```python
from build123d import *

# Parameters (mm, degrees)
F0_R     = 2.65
F0_R_2   = 3.15
F1_DEPTH = 5
F2_R     = 4
F3_R     = 3


with BuildPart() as f1:
    # F0 (on Top) → F1 (new body)
    with BuildSketch(Plane.XY):
        with BuildLine():
            ThreePointArc((-30, -20), (0, -14.852814), (30, -20))
            ThreePointArc((30, -20), (26.568542, 0), (30, 20))
            ThreePointArc((30, 20), (0, 14.852814), (-30, 20))
            ThreePointArc((-30, 20), (-26.568542, 0), (-30, -20))
        make_face()
        with Locations((-20, -10)):
            Circle(F0_R, mode=Mode.SUBTRACT)
        with Locations((20, -10)):
            Circle(F0_R, mode=Mode.SUBTRACT)
        with Locations((-20, 10)):
            Circle(F0_R_2, mode=Mode.SUBTRACT)
        Polygon((10, 0), (5, -8.660254), (-5, -8.660254), (-10, 0), (-5, 8.660254), (5, 8.660254), align=None, mode=Mode.SUBTRACT)
        with Locations((20, 10)):
            Circle(F0_R_2, mode=Mode.SUBTRACT)
    extrude(amount=F1_DEPTH)

    # F2
    f2_edges = [f1.edges().sort_by_distance(p)[0] for p in [
        (30, 20, 2.5),
        (-30, 20, 2.5),
        (-30, -20, 2.5),
        (30, -20, 2.5),
    ]]
    fillet(f2_edges, radius=F2_R)

    # F3
    f3_edges = [f1.edges().sort_by_distance(p)[0] for p in [
        (5, 8.660254, 2.5),
        (-5, 8.660254, 2.5),
        (10, 0, 2.5),
        (5, -8.660254, 2.5),
        (-5, -8.660254, 2.5),
        (-10, 0, 2.5),
    ]]
    fillet(f3_edges, radius=F3_R)


solid = f1.part
```
Verification items for the finished model (mm, model axes). A direction names the side the tool comes from. Coordinates: 2 decimals unless noted, no trailing zeros. Write each loop counter-clockwise with the first axis right and the second up, starting at its lowest first coordinate (ties: lowest second). Pieces come first, ordered by that corner, then holes. Notation, with made-up numbers: M 83.25,-17.75 L 115.25,-17.75 A15 cw 115.25,2.25 Z; hole C 17.25,73.5 d1. An arc over 180 degrees is marked long. One line per item, written item: value.
Item 1: Section check A-A, the plane x = -4. Record the boundary of the cut face in (y, z).
Check sheet entries:
outline: M -14.94,0 L -8.57,0 L -8.57,5 L -14.94,5 Z; M 8.57,0 L 14.94,0 L 14.94,5 L 8.57,5 Z
Item 2: Mould release check, pull along Y, two halves, no side actions. Record for faces 3 (the cylindrical face through (0.327, 14.853, 2.465)), 4 (the cylindrical face through (-4.75, -8.27, 2.54)), 5 (the flat face through (6, -8, 5)): pulls with the +Y half, pulls with the -Y half, needs draft (parallel to the pull), parting line crosses it, or undercut.
Check sheet entries:
face 3: pulls with the +Y half
face 4: undercut
face 5: needs draft
Item 3: Section check D-D, the plane x = 21.5. Record the boundary of the cut face in (y, z).
Check sheet entries:
outline: M -17.46,0 L -12.18,0 L -12.18,5 L -17.46,5 Z; M -7.82,0 L 7.23,0 L 7.23,5 L -7.82,5 Z; M 12.77,0 L 17.46,0 L 17.46,5 L 12.77,5 Z
Item 4: Section check C-C, the plane y = 10. Record the boundary of the cut face in (x, z), plus the area to 3 significant figures.
Check sheet entries:
outline: M -27.41,0 L -23.15,0 L -23.15,5 L -27.41,5 Z; M -16.85,0 L 16.85,0 L 16.85,5 L -16.85,5 Z; M 23.15,0 L 27.41,0 L 27.41,5 L 23.15,5 Z
area: 211 mm^2
Item 5: Scan lines: line 1 along Y through (x, z) = (-22, 4.65); line 2 along Y through (x, z) = (-20, 2.75); line 3 along Y through (x, z) = (24, 3.2). Record each from-to range of solid material in increasing order.
Check sheet entries:
line 1: y = -17.58 to -11.74, -8.26 to 7.57, 12.43 to 17.58
line 2: y = -17.1 to -12.65, -7.35 to 6.85, 13.15 to 17.1
line 3: y = -18 to 18
Item 6: Gauge pin test, flat end, axial feed: pin 1 Ø4 at (x, y) = (-20, 10) entering from +Z. Record the tip position at first contact, or that the pin passes through.
Check sheet entries:
pin 1: passes through
Item 7: Section check B-B, the plane y = -8. Record the boundary of the cut face in (x, z).
Check sheet entries:
outline: M -27.1,0 L -21.74,0 L -21.74,5 L -27.1,5 Z; M -18.26,0 L -5.15,0 L -5.15,5 L -18.26,5 Z; M 5.15,0 L 18.26,0 L 18.26,5 L 5.15,5 Z; M 21.74,0 L 27.1,0 L 27.1,5 L 21.74,5 Z
Item 8: Access from +Z, -Z, +X, -X, +Y, -Y to the whole of each face (thin tool, end or side, straight path). Record for faces 1 (the cylindrical face through (-9.536, 0.022, 2.535)), 2 (the flat face through (6, -8, 0)).
Check sheet entries:
face 1: +Z, -Z
face 2: -Z, +X, -X, +Y, -Y
